from build123d import *

# Parameters (mm, degrees)
ESQUISSE1_W        = 5.6
ESQUISSE1_H        = 36.8
ESQUISSE1_W_2      = 2.6
ESQUISSE1_H_2      = 31.8
BOSS_EXTRU_1_DEPTH = 20
CONG_1_R           = 2


with BuildPart() as part:
    # Esquisse1 → Boss.-Extru.1 (new body)
    with BuildSketch(Plane.XY):
        with Locations((0.188649611, -11.438461538)):
            Rectangle(ESQUISSE1_W, ESQUISSE1_H)
        with Locations((0.188649611, -11.438461538)):
            Rectangle(ESQUISSE1_W_2, ESQUISSE1_H_2, mode=Mode.SUBTRACT)
    extrude(amount=BOSS_EXTRU_1_DEPTH)

    # Congé1
    cong_1_edges = [part.edges().sort_by_distance(p)[0] for p in [
        (-2.611350389, 6.961538462, 10),
        (2.988649611, 6.961538462, 10),
        (2.988649611, -29.838461538, 10),
        (-2.611350389, -29.838461538, 10),
    ]]
    fillet(cong_1_edges, radius=CONG_1_R)


solid = part.part
Could you check a few things on this model? Use its own coordinates, in mm. A direction names the side the tool comes from. Round coordinates to 2 decimals unless told otherwise and drop trailing zeros. Write each loop counter-clockwise with the first axis right and the second up, starting at its lowest first coordinate (ties: lowest second). Pieces come first, ordered by that corner, then holes. Notation, with made-up numbers: (11, -28.5) -> (63, -28.5) arc R27 cw to (63, 4.5) -> close; hole circle Ø1 at (-37.5, 53). An arc over 180 degrees is marked (long way). Use a Markdown table: item, result.
1. Please list where these lines run through material, in increasing order: probe 1 along X at (y, z) = (1.5, 17); probe 2 along Y at (x, z) = (0.5, 1); probe 3 along Y at (x, z) = (1.3, 4.5).
Answer key:
| item | result |
|---|---|
| probe 1 | x = -2.61 to -1.11, 1.49 to 2.99 |
| probe 2 | y = -29.84 to -27.34, 4.46 to 6.96 |
| probe 3 | y = -29.81 to -27.34, 4.46 to 6.94 |
2. We'd pull the mould along X, two halves only. Please class faces 1 (the face through (2.387, -29.268, 10.14)), 2 (the face through (-1.111, -12, 10)), 3 (the face through (-2, 6.4, 10.1)): +X half, -X half, draft (parallel to the pull), parting line (faces both ways), or undercut.
Answer key:
| item | result |
|---|---|
| face 1 | +X half |
| face 2 | undercut |
| face 3 | -X half |
3. If we section it at A-A (x = -0.2): List the corners of the cut face in (y, z) for me, then the cut area to 4 significant figures.
Answer key:
| item | result |
|---|---|
| outline | (-29.84, 0) -> (-27.34, 0) -> (-27.34, 20) -> (-29.84, 20) -> close; (4.46, 0) -> (6.96, 0) -> (6.96, 20) -> (4.46, 20) -> close |
| area | 100.0 mm^2 |
4. If we section it at C-C (z = 1.75): List the corners of the cut face in (x, y) for me, then the cut area to 3 significant figures.
Answer key:
| item | result |
|---|---|
| outline | (-2.61, -27.84) arc R2 ccw to (-0.61, -29.84) -> (0.99, -29.84) arc R2 ccw to (2.99, -27.84) -> (2.99, 4.96) arc R2 ccw to (0.99, 6.96) -> (-0.61, 6.96) arc R2 ccw to (-2.61, 4.96) -> close; hole (-1.11, -27.34) -> (1.49, -27.34) -> (1.49, 4.46) -> (-1.11, 4.46) -> close |
| area | 120 mm^2 |
5. Which directions (+Z, -Z, +X, -X, +Y, -Y) give clear straight access to the entire face, cutting with the end or side of a thin tool? Please do faces 4 (the face through (2.39, 6.39, 10.14)), 5 (the face through (0, -27.338, 10)).
Answer key:
| item | result |
|---|---|
| face 4 | +Z, -Z, +X, +Y |
| face 5 | +Z, -Z |
6. If we section it at B-B (y = -8): List the corners of the cut face in (x, z) for me, then the cut area to 3 significant figures.
Answer key:
| item | result |
|---|---|
| outline | (-2.61, 0) -> (-1.11, 0) -> (-1.11, 20) -> (-2.61, 20) -> close; (1.49, 0) -> (2.99, 0) -> (2.99, 20) -> (1.49, 20) -> close |
| area | 60.0 mm^2 |
7. If we section it at D-D (x = 2.3): List the corners of the cut face in (y, z) for me.
Answer key:
| item | result |
|---|---|
| outline | (-29.35, 0) -> (6.47, 0) -> (6.47, 20) -> (-29.35, 20) -> close |
